Geometry: final body of the model. Coordinates: model frame, mm. Face numbers are marked on the shaded views. A direction names the side the tool comes from. Round coordinates to 2 decimals unless told otherwise and drop trailing zeros. Loops run counter-clockwise (first coordinate to the right, second up) from the corner with the lowest first, then second, coordinate; pieces in that order, holes last. Notation, with made-up numbers: M 59,-36.75 L 65,-36.75 A26 ccw 65,-6.75 Z; hole C 16,-3.75 d4. An arc over 180 degrees is marked long. Write each question's results on one line, items separated by ' | '.
```python
from build123d import *

# Parameters (mm, degrees)
SKETCH1_W                                        = 26
SKETCH1_H                                        = 12
BOSS_EXTRUDE1_DEPTH                              = 9
CUT_EXTRUDE1_DEPTH                               = 40.217343102
CBORE_FOR_M4_HEX_HEAD_MACHINE_SCREW1_D           = 4.5
CBORE_FOR_M4_HEX_HEAD_MACHINE_SCREW1_CBORE_D     = 8
CBORE_FOR_M4_HEX_HEAD_MACHINE_SCREW1_CBORE_DEPTH = 4.5


with BuildPart() as part:
    # Sketch1 → Boss-Extrude1 (new body)
    with BuildSketch(Plane(origin=(0, 35, 0), x_dir=(1, 0, 0), z_dir=(0, 1, 0))):
        Rectangle(SKETCH1_W, SKETCH1_H)
    extrude(amount=-BOSS_EXTRUDE1_DEPTH)

    # Sketch2 → Cut-Extrude1 (cut, through all)
    with BuildSketch(Plane(origin=(0, 0, -6), x_dir=(-1, 0, 0), z_dir=(0, 0, -1))):
        with BuildLine():
            Line((-4.656329697, 26), (4.656329697, 26))
            ThreePointArc((4.656329697, 26), (0, 29.7625), (-4.656329697, 26))
        make_face()
    extrude(amount=-CUT_EXTRUDE1_DEPTH, mode=Mode.SUBTRACT)

    # CBORE for M4 Hex Head Machine Screw1 (through all)
    with Locations(Plane(origin=(0, 35, 0), x_dir=(1, 0, 0), z_dir=(0, 1, 0))):
        with Locations((-8, 0), (8, 0)):
            CounterBoreHole(CBORE_FOR_M4_HEX_HEAD_MACHINE_SCREW1_D / 2, CBORE_FOR_M4_HEX_HEAD_MACHINE_SCREW1_CBORE_D / 2, CBORE_FOR_M4_HEX_HEAD_MACHINE_SCREW1_CBORE_DEPTH)


solid = part.part
```
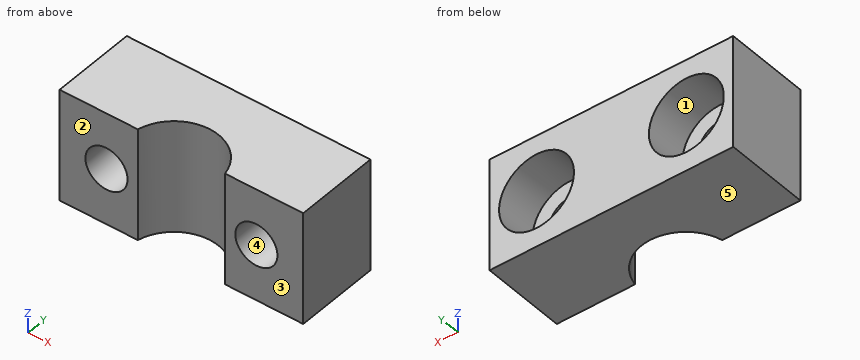
1. Section C-C (y = 28). Output: boundary loops of the cut face in (x, z).
Answer key:
outline: M -13,-6 L -3.7,-6 L -3.7,6 L -13,6 Z; M 3.7,-6 L 13,-6 L 13,6 L 3.7,6 Z; hole C -8,0 d4.5; hole C 8,0 d4.5
2. Section A-A (x = -8). Output: boundary loops of the cut face in (y, z).
Answer key:
outline: M 26,-6 L 35,-6 L 35,-4 L 30.5,-4 L 30.5,-2.25 L 26,-2.25 Z; M 26,2.25 L 30.5,2.25 L 30.5,4 L 35,4 L 35,6 L 26,6 Z
3. Section D-D (y = 32.25). Output: boundary loops of the cut face in (x, z).
Answer key:
outline: M -13,-6 L 13,-6 L 13,6 L -13,6 Z; hole C -8,0 d8; hole C 8,0 d8
4. Section B-B (z = 0). Count the separate pieces of the cut face and the enclosed holes in it, then the cut area to 3 significant figures.
Answer key:
separate pieces: 3 | enclosed holes: 0 | area: 95.3 mm²
5. Access query for the marked faces 1 and 2. Directions: +Z, -Z, +X, -X, +Y, -Y. A direction counts if a zero-diameter tool reaches every point of the face in a straight line with its end or side. Return the directions, or none.
Answer key:
face 1: +Y | face 2: +Z, -Z, +X, -X, -Y
6. Draft query along Z for the marked faces 3, 4 and 5. Return one class per face: pulls with the +Z half, pulls with the -Z half, needs draft (parallel to the pull), parting line crosses it, or undercut.
Answer key:
face 3: needs draft | face 4: undercut | face 5: pulls with the -Z half
7. Pin query (flat end, axial travel): P1, Ø6, axis at x = -8, z = 0, coming from the +Y side. Return the tip coordinate at first contact, or that it passes through.
Answer key:
P1: stops at y = 30.5
8. Ray query, probe 1 along Z at (x, y) = (-8, 29.2); probe 2 along X at (y, z) = (34.75, -2.25); probe 3 along Z at (x, y) = (-8, 34.15). Return the intervals inside material, ascending.
Answer key:
probe 1: z = -6 to -2.25, 2.25 to 6 | probe 2: x = -13 to -11.31, -4.69 to 4.69, 11.31 to 13 | probe 3: z = -6 to -4, 4 to 6
